Source: CAD feature listing. Evaluate the final solid. Frame: model axes, mm. Give positions to 0.01 mm unless a question says otherwise; leave off trailing zeros. Loops run counter-clockwise (first coordinate to the right, second up) from the corner with the lowest first, then second, coordinate; pieces in that order, holes last. Notation, with made-up numbers: M 67.5,28 L 121.5,28 A17 ccw 121.5,48 Z; hole C -39,63 d9. An arc over 180 degrees is marked long. Write item = value, one per line.
from build123d import *

# Parameters (mm, degrees)
ESBO_O1_R                = 8.5
RESSALTO_EXTRUS_O1_DEPTH = 1


with BuildPart() as part:
    # Esboço1 → Ressalto-extrusão1 (new body)
    with BuildSketch(Plane.XY):
        Circle(ESBO_O1_R)
        with BuildLine():
            Line((-0.654508497, 0.475528258), (-4.90223967, 6.322028647))
            ThreePointArc((-4.90223967, 6.322028647), (-6.472135955, 4.702282018), (-7.52748191, 2.708692692))
            Line((-7.52748191, 2.708692692), (-0.654508497, 0.475528258))
        make_face(mode=Mode.SUBTRACT)
        with BuildLine():
            Line((-0.25, 0.769420884), (-0.25, 7.996092796))
            ThreePointArc((-0.25, 7.996092796), (-2.472135955, 7.60845213), (-4.497731173, 6.615921274))
            Line((-4.497731173, 6.615921274), (-0.25, 0.769420884))
        make_face(mode=Mode.SUBTRACT)
        with BuildLine():
            Line((0.25, 0.769420884), (4.497731173, 6.615921274))
            ThreePointArc((4.497731173, 6.615921274), (2.472135955, 7.60845213), (0.25, 7.996092796))
            Line((0.25, 7.996092796), (0.25, 0.769420884))
        make_face(mode=Mode.SUBTRACT)
        with BuildLine():
            Line((0.654508497, 0.475528258), (7.52748191, 2.708692692))
            ThreePointArc((7.52748191, 2.708692692), (6.472135955, 4.702282018), (4.90223967, 6.322028647))
            Line((4.90223967, 6.322028647), (0.654508497, 0.475528258))
        make_face(mode=Mode.SUBTRACT)
        with BuildLine():
            Line((0.809016994, 0), (7.681990407, -2.233164433))
            ThreePointArc((7.681990407, -2.233164433), (8, 0), (7.681990407, 2.233164433))
            Line((7.681990407, 2.233164433), (0.809016994, 0))
        make_face(mode=Mode.SUBTRACT)
        with BuildLine():
            Line((0.654508497, -0.475528258), (4.90223967, -6.322028647))
            ThreePointArc((4.90223967, -6.322028647), (6.472135955, -4.702282018), (7.52748191, -2.708692692))
            Line((7.52748191, -2.708692692), (0.654508497, -0.475528258))
        make_face(mode=Mode.SUBTRACT)
        with BuildLine():
            Line((0.25, -0.769420884), (0.25, -7.996092796))
            ThreePointArc((0.25, -7.996092796), (2.472135955, -7.60845213), (4.497731173, -6.615921274))
            Line((4.497731173, -6.615921274), (0.25, -0.769420884))
        make_face(mode=Mode.SUBTRACT)
        with BuildLine():
            Line((-0.25, -0.769420884), (-4.497731173, -6.615921274))
            ThreePointArc((-4.497731173, -6.615921274), (-2.472135955, -7.60845213), (-0.25, -7.996092796))
            Line((-0.25, -7.996092796), (-0.25, -0.769420884))
        make_face(mode=Mode.SUBTRACT)
        with BuildLine():
            Line((-0.654508497, -0.475528258), (-7.52748191, -2.708692692))
            ThreePointArc((-7.52748191, -2.708692692), (-6.472135955, -4.702282018), (-4.90223967, -6.322028647))
            Line((-4.90223967, -6.322028647), (-0.654508497, -0.475528258))
        make_face(mode=Mode.SUBTRACT)
        with BuildLine():
            Line((-0.809016994, 0), (-7.681990407, 2.233164433))
            ThreePointArc((-7.681990407, 2.233164433), (-8, 0), (-7.681990407, -2.233164433))
            Line((-7.681990407, -2.233164433), (-0.809016994, 0))
        make_face(mode=Mode.SUBTRACT)
    extrude(amount=RESSALTO_EXTRUS_O1_DEPTH)


solid = part.part
1. Cut plane C-C, the plane x = 2.5. Return the cut outline in (y, z).
Derived:
outline = M -8.12,0 L -7.6,0 L -7.6,1 L -8.12,1 Z; M -3.87,0 L -3.02,0 L -3.02,1 L -3.87,1 Z; M -1.08,0 L -0.55,0 L -0.55,1 L -1.08,1 Z; M 0.55,0 L 1.08,0 L 1.08,1 L 0.55,1 Z; M 3.02,0 L 3.87,0 L 3.87,1 L 3.02,1 Z; M 7.6,0 L 8.12,0 L 8.12,1 L 7.6,1 Z
2. Material intervals for probe 1 along X at (y, z) = (-5.25, 0.7); probe 2 along X at (y, z) = (3.25, 0.4); probe 3 along Y at (x, z) = (-6.5, 0.95), sorted ascending. Write a range as from..to.
Derived:
probe_1 = -6.68..-6.04, -4.12..-3.51, -0.25..0.25, 3.51..4.12, 6.04..6.68
probe_2 = -7.85..-7.31, -2.67..-2.05, -0.25..0.25, 2.05..2.67, 7.31..7.85
probe_3 = -5.48..-4.66, -2.37..-1.85, 1.85..2.37, 4.66..5.48
3. Pull-direction query (X, two-part tool) for faces 1 (the flat face through (-4.2, 1.1, 0.5)), 2 (the cylindrical face through (4.57, 7.167, 0.493)), 3 (the flat face through (0, -1, 1)); classes: +X half, -X half, draft (parallel to the pull), parting line (faces both ways), or undercut.
Derived:
face_1 = undercut
face_2 = parting line
face_3 = draft
4. Cut plane D-D, the plane y = -4. Return the cut outline in (x, z), then the cut area to 3 significant figures.
Derived:
outline = M -7.5,0 L -6.93,0 L -6.93,1 L -7.5,1 Z; M -3.22,0 L -2.6,0 L -2.6,1 L -3.22,1 Z; M -0.25,0 L 0.25,0 L 0.25,1 L -0.25,1 Z; M 2.6,0 L 3.22,0 L 3.22,1 L 2.6,1 Z; M 6.93,0 L 7.5,0 L 7.5,1 L 6.93,1 Z
area = 2.88 mm²
5. Cut plane A-A, the plane z = 0.35. Count the separate pieces of the cut face and the enclosed holes in it, then the cut area to 3 significant figures.
Derived:
separate_pieces = 1
enclosed_holes = 10
area = 64.0 mm²
6. Cut plane B-B, the plane y = 1.75. Return the cut outline in (x, z), then the cut area to 3 significant figures.
Derived:
outline = M -8.32,0 L -7.81,0 L -7.81,1 L -8.32,1 Z; M -6.19,0 L -4.58,0 L -4.58,1 L -6.19,1 Z; M -1.58,0 L -0.96,0 L -0.96,1 L -1.58,1 Z; M -0.25,0 L 0.25,0 L 0.25,1 L -0.25,1 Z; M 0.96,0 L 1.58,0 L 1.58,1 L 0.96,1 Z; M 4.58,0 L 6.19,0 L 6.19,1 L 4.58,1 Z; M 7.81,0 L 8.32,0 L 8.32,1 L 7.81,1 Z
area = 6.00 mm²
